The listing builds one solid part. Answer for the finished solid, in the listing's coordinates (mm). A direction names the side the tool comes from. Give positions to 0.01 mm unless a question says otherwise; leave off trailing zeros. Order: outer loops, then holes, each group sorted by start corner. A loop starts at its lowest first (then second) coordinate and runs counter-clockwise, first axis right, second up. Notation, with made-up numbers: (-24, 21) - (-20, 21) arc R11 cw to (-20, 26) - close; hole circle Ø1 at (56, -31). An arc over 180 degrees is marked (long way). Use a Markdown table: item, result. Add a question column.
1) Flat-ended cylindrical pins translate along their axes: pin 1 (2 mm diameter, centred on x = 13, y = 3, fed in from -Z); pin 2 (2 mm diameter, centred on x = 0, z = -10, fed in from +Y); pin 3 (2 mm diameter, centred on y = 2, z = -3.5, fed in from -X). Find the tip coordinate at first contact, or state that the pin passes through.
2) Find section C-C, the plane x = -12.5. Determine the outline of the cut face in (y, z), plus the area to 3 significant figures.
3) Find section B-B, the plane z = 2. Determine the outline of the cut face in (x, y).
4) Straight lines are drawn through the part: line 1 (Z direction, x = 0, y = 5.8); line 2 (Z direction, x = 0, y = 5.25); line 3 (Y direction, x = 5, z = 14.5). For each, find the intervals that lie inside material, in ascending order.
5) Find section D-D, the plane y = 6.5. Determine the outline of the cut face in (x, z), plus the area to 4 significant figures.
6) For faces 1 (the face through (-3, 7, -3)), 2 (the face through (4, 8.5, 4)), 3 (the face through (-0.273, 5.542, -11.082)), determine the directions among +Z, -Z, +X, -X, +Y, -Y from which every point of the face is accessible in a straight line to the end or side of a thin tool.
7) Find section A-A, the plane x = 0. Determine the outline of the cut face in (y, z), plus the area to 3 significant figures.
8) The mould has two halves that part along X. Classify faces 4 (the face through (9.139, 6.979, -14.334)), 5 (the face through (-0.273, 5.542, 6.918)), 6 (the face through (2.4, 3.5, -4.5)), 7 (the face through (6, 5.5, 14)): released by +X, released by -X, zero draft, split by the parting line, or undercut.
from build123d import *

# Parameters (mm, degrees)
SKETCH1_R           = 15
BOSS_EXTRUDE1_DEPTH = 5.5
SKETCH2_R           = 17
BOSS_EXTRUDE2_DEPTH = 3
SKETCH3_R           = 5.1
CUT_EXTRUDE1_DEPTH  = 7
SKETCH4_R           = 2.1
SKETCH4_R_2         = 4
CUT_EXTRUDE2_DEPTH  = 6


with BuildPart() as part:
    # Sketch1 → Boss-Extrude1 (new body)
    with BuildSketch(Plane(origin=(0, 0, 0), x_dir=(1, 0, 0), z_dir=(0, 1, 0))):
        Circle(SKETCH1_R)
    extrude(amount=BOSS_EXTRUDE1_DEPTH)

    # Sketch2 → Boss-Extrude2 (add)
    with BuildSketch(Plane(origin=(0, 5.5, 0), x_dir=(1, 0, 0), z_dir=(0, 1, 0))):
        Circle(SKETCH2_R)
    extrude(amount=BOSS_EXTRUDE2_DEPTH)

    # Sketch3 → Cut-Extrude1 (cut)
    with BuildSketch(Plane.XZ):
        Circle(SKETCH3_R)
    extrude(amount=-CUT_EXTRUDE1_DEPTH, mode=Mode.SUBTRACT)

    # Sketch4 → Cut-Extrude2 (cut)
    with BuildSketch(Plane(origin=(0, 8.5, 0), x_dir=(1, 0, 0), z_dir=(0, 1, 0))):
        with Locations((0, 9)):
            Circle(SKETCH4_R)
        with Locations((0, -9)):
            Circle(SKETCH4_R)
        Circle(SKETCH4_R_2)
    extrude(amount=-CUT_EXTRUDE2_DEPTH, mode=Mode.SUBTRACT)


solid = part.part
The answers:
| question | item | result |
|---|---|---|
| 1 | pin 1 | z = -9 |
| 1 | pin 2 | y = 2.5 |
| 1 | pin 3 | x = -14.79 |
| 2 | outline | (0, -8.29) - (5.5, -8.29) - (5.5, -11.52) - (8.5, -11.52) - (8.5, 11.52) - (5.5, 11.52) - (5.5, 8.29) - (0, 8.29) - close |
| 2 | area | 160 mm2 |
| 3 | outline | (-16.88, 5.5) - (-14.87, 5.5) - (-14.87, 0) - (-4.69, 0) - (-4.69, 7) - (-3.46, 7) - (-3.46, 8.5) - (-16.88, 8.5) - close; (3.46, 7) - (4.69, 7) - (4.69, 0) - (14.87, 0) - (14.87, 5.5) - (16.88, 5.5) - (16.88, 8.5) - (3.46, 8.5) - close |
| 4 | line 1 | -17 to -11.1, -6.9 to -5.1, 5.1 to 6.9, 11.1 to 17 |
| 4 | line 2 | -15 to -11.1, -6.9 to -5.1, 5.1 to 6.9, 11.1 to 15 |
| 4 | line 3 | 5.5 to 8.5 |
| 5 | outline | circle Ø34 at (0, 0); hole circle Ø10.2 at (0, 0); hole circle Ø4.2 at (0, -9); hole circle Ø4.2 at (0, 9) |
| 5 | area | 798.5 mm2 |
| 6 | face 1 | -Y |
| 6 | face 2 | +Z, -Z, +X, -X, +Y |
| 6 | face 3 | +Y |
| 7 | outline | (0, -15) - (5.5, -15) - (5.5, -17) - (8.5, -17) - (8.5, -11.1) - (2.5, -11.1) - (2.5, -6.9) - (8.5, -6.9) - (8.5, -4) - (7, -4) - (7, -5.1) - (0, -5.1) - close; (0, 5.1) - (7, 5.1) - (7, 4) - (8.5, 4) - (8.5, 6.9) - (2.5, 6.9) - (2.5, 11.1) - (8.5, 11.1) - (8.5, 17) - (5.5, 17) - (5.5, 15) - (0, 15) - close |
| 7 | area | 133 mm2 |
| 8 | face 4 | split by the parting line |
| 8 | face 5 | undercut |
| 8 | face 6 | undercut |
| 8 | face 7 | zero draft |
